```python
from build123d import *

# Parameters (mm, degrees)
SKETCH1_W               = 12.7
SKETCH1_H               = 38.1
BOSS_EXTRUDE1_DEPTH     = 6.35
CUT_EXTRUDE1_DEPTH      = 41.659838908
CUT_EXTRUDE1_DEPTH_BACK = 41.659838908
SKETCH2_R               = 3.81


with BuildPart() as part:
    # Sketch1 → Boss-Extrude1 (new body)
    with BuildSketch(Plane.XY):
        with Locations((6.35, -19.05)):
            Rectangle(SKETCH1_W, SKETCH1_H)
    extrude(amount=BOSS_EXTRUDE1_DEPTH)

    # Sketch2 → Cut-Extrude1 (cut, two sides: drawn at the far end of the back side and taken through both)
    with BuildSketch(Plane.XY.offset(6.35).offset(-CUT_EXTRUDE1_DEPTH_BACK)):
        with Locations((6.35, -6.35)):
            Circle(SKETCH2_R)
    extrude(amount=CUT_EXTRUDE1_DEPTH + CUT_EXTRUDE1_DEPTH_BACK, mode=Mode.SUBTRACT)


solid = part.part
```
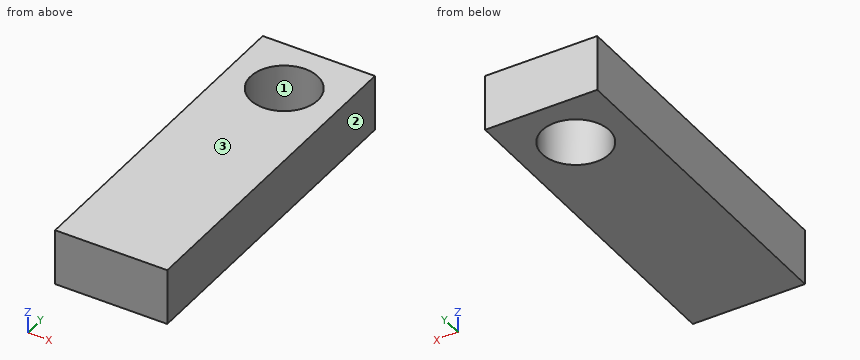
For this review, take the finished solid that the model builds, in its own axes (mm). Face numbers are marked on the shaded views. Coordinates: 2 decimals unless noted, no trailing zeros. Write each loop counter-clockwise with the first axis right and the second up, starting at its lowest first coordinate (ties: lowest second). Pieces come first, ordered by that corner, then holes. Notation, with made-up numbers: (26, -21) - (64, -21) arc R27 cw to (64, 15) - close; hole circle Ø8 at (65.25, -18.5). An arc over 180 degrees is marked (long way). Answer in a Markdown table with one row per item. Add a question column.
Q1. Draft analysis for pull direction X (two halves, no side actions). For the marked faces 1, 2 and 3, state which applies: +X half, -X half, draft (parallel to the pull), parting line (faces both ways), or undercut.
Q2. We need section C-C, the plane z = 0.75. State the section outline as (x, y) points.
Q3. We need section B-B, the plane x = 6.35. State the section outline as (y, z) points.
Q4. We need section A-A, the plane y = -6.35. State the section outline as (x, z) points, and give its area (3 significant figures).
Q5. For probe 1 along Y at (x, z) = (6.35, 2.5); probe 2 along X at (y, z) = (-6.35, 3.25); probe 3 along X at (y, z) = (-5, 3.75), list the stretches that pass through material, from the lowest coordinate up.
Answer list:
| question | item | result |
|---|---|---|
| 1 | face 1 | undercut |
| 1 | face 2 | +X half |
| 1 | face 3 | draft |
| 2 | outline | (0, -38.1) - (12.7, -38.1) - (12.7, 0) - (0, 0) - close; hole circle Ø7.62 at (6.35, -6.35) |
| 3 | outline | (-38.1, 0) - (-10.16, 0) - (-10.16, 6.35) - (-38.1, 6.35) - close; (-2.54, 0) - (0, 0) - (0, 6.35) - (-2.54, 6.35) - close |
| 4 | outline | (0, 0) - (2.54, 0) - (2.54, 6.35) - (0, 6.35) - close; (10.16, 0) - (12.7, 0) - (12.7, 6.35) - (10.16, 6.35) - close |
| 4 | area | 32.3 mm2 |
| 5 | probe 1 | y = -38.1 to -10.16, -2.54 to 0 |
| 5 | probe 2 | x = 0 to 2.54, 10.16 to 12.7 |
| 5 | probe 3 | x = 0 to 2.79, 9.91 to 12.7 |
